from build123d import *

# Parameters (mm, degrees)
FILLET_1_R          = 0.2
CUT_EXTRUDE_1_DEPTH = 1.5


with BuildPart() as part:
    # 草图1 → 旋转1 (revolve)
    with BuildSketch(Plane(origin=(0, 0, 0), x_dir=(0, 0, -1), z_dir=(1, 0, 0))):
        Polygon((0, 0), (-2.25, 0), (-2.25, 3), (-1.5, 3), (-1.5, 38), (0, 38), align=None)
    revolve(axis=Axis((0, 38, 0), (0, -1, 0)))

    # 圆角1
    fillet_1_edges = [part.edges().sort_by_distance(p)[0] for p in [
        (0, 3, -1.5),
    ]]
    fillet(fillet_1_edges, radius=FILLET_1_R)

    # 草图2 → 切除-拉伸1 (cut)
    with BuildSketch(Plane.XZ):
        Polygon((0, 1.35099963), (-1.17, 0.675499815), (-1.17, -0.675499815), (0, -1.35099963), (1.17, -0.675499815), (1.17, 0.675499815), align=None)
    extrude(amount=-CUT_EXTRUDE_1_DEPTH, mode=Mode.SUBTRACT)


solid = part.part
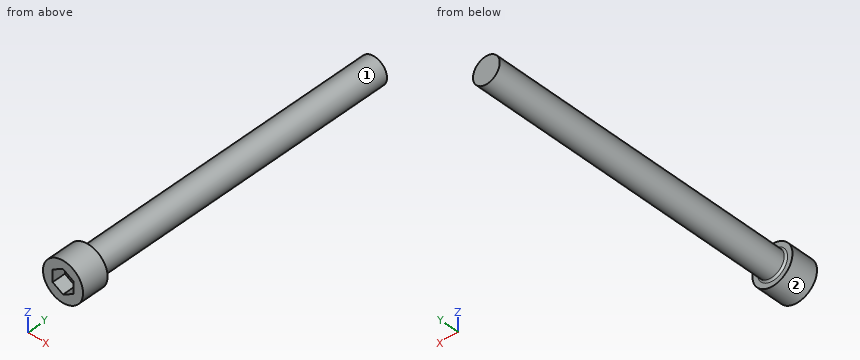
The model under review builds one solid part; all positions refer to its coordinate system, in mm. Face numbers are marked on the shaded views. A direction names the side the tool comes from. Round coordinates to 2 decimals unless told otherwise and drop trailing zeros. Order: outer loops, then holes, each group sorted by start corner. A loop starts at its lowest first (then second) coordinate and runs counter-clockwise, first axis right, second up. Notation, with made-up numbers: (-7.5, 9.5) -> (8.5, 9.5) arc R19 cw to (8.5, 46.5) -> close; hole circle Ø8 at (26, 4.25). An arc over 180 degrees is marked (long way). Return JSON: item names as keys, results as strings.
1. Take a section at B-B (y = 33). Write out the cut boundary in (x, z).
Answer block:
{"outline": "circle Ø3 at (0, 0)"}
2. For the marked faces 1 and 2, list the 3-axis set-ups (+Z, -Z, +X, -X, +Y, -Y) from which the entire face can be reached by the end or side of a thin tool; tool diameter is ignored.
Answer block:
{"face 1": "+Y", "face 2": "+Y, -Y"}
3. Insertion check: P1, Ø1, axis at y = 27, z = -0.5, coming from the -X side; P2, Ø2.5, axis at x = 0, z = -0.5, coming from the -Y side; P3, Ø1, axis at x = -0.5, y = 24.5, coming from the -Z side. Each pin has a flat end and moves straight along its axis. Give the tip position at first contact, or say it passes through.
Answer block:
{"P1": "stops at x = -1.5", "P2": "stops at y = 0", "P3": "stops at z = -1.5"}
4. Take a section at A-A (z = 0). Write out the cut boundary in (x, y), then the cut area to 3 significant figures.
Answer block:
{"outline": "(-2.25, 0) -> (-1.17, 0) -> (-1.17, 1.5) -> (1.17, 1.5) -> (1.17, 0) -> (2.25, 0) -> (2.25, 3) -> (1.7, 3) arc R0.2 cw to (1.5, 3.2) -> (1.5, 38) -> (-1.5, 38) -> (-1.5, 3.2) arc R0.2 cw to (-1.7, 3) -> (-2.25, 3) -> close", "area": "115 mm²"}
5. For L1, parallel to Z at x = 0.05, y = 28; L2, parallel to Y at x = 0.7, z = -2, list the stretches that pass through material, from the lowest coordinate up. Write a range as [from, to].
Answer block:
{"L1": "z = [-1.5, 1.5]", "L2": "y = [0, 3]"}
